Build history of the part. All positions in model axes, mm. A direction names the side the tool comes from. Coordinates: 2 decimals unless noted, no trailing zeros. Order: outer loops, then holes, each group sorted by start corner. A loop starts at its lowest first (then second) coordinate and runs counter-clockwise, first axis right, second up. Notation, with made-up numbers: (-23.5, 58.5) -> (11.5, 58.5) arc R23 cw to (11.5, 76.5) -> close; hole circle Ø6 at (-12.75, 4.25). An arc over 180 degrees is marked (long way). Write each question's results on one line, items separated by ' | '.
from build123d import *

# Parameters (mm, degrees)
SKETCH003_R        = 38.1
PAD003_DEPTH       = 2
SKETCH004_R        = 8
PAD004_DEPTH       = 16
SKETCH005_R        = 38.1
PAD005_DEPTH       = 2
POCKET_DEPTH       = 239.207569
POLARPATTERN_COUNT = 3
SKETCH007_R        = 4
POCKET001_DEPTH    = 20.001


with BuildPart() as part:
    # Sketch003 → Pad003 (new body)
    with BuildSketch(Plane.XY):
        Circle(SKETCH003_R)
    extrude(amount=PAD003_DEPTH)

    # Sketch004 (on Face3 of Pad003) → Pad004 (join)
    with BuildSketch(Plane.XY.offset(2)):
        Circle(SKETCH004_R)
    extrude(amount=PAD004_DEPTH)

    # Sketch005 (on Face5 of Pad004) → Pad005 (join)
    with BuildSketch(Plane.XY.offset(18)):
        Circle(SKETCH005_R)
    extrude(amount=PAD005_DEPTH)

    # Sketch006 (on Face3 of Pad005) → Pocket (cut, through all)
    with BuildSketch(Plane.XY.offset(20)):
        with BuildLine():
            Line((-15, 29.1), (15, 29.1))
            ThreePointArc((15.842922, 27.561965), (15.876937, 28.580606), (15, 29.1))
            Line((15.842922, 27.561965), (6.842922, 13.461965))
            ThreePointArc((6, 13), (6.480606, 13.123063), (6.842922, 13.461965))
            Line((6, 13), (-6, 13))
            ThreePointArc((-6.842922, 13.461965), (-6.480606, 13.123063), (-6, 13))
            Line((-6.842922, 13.461965), (-15.842922, 27.561965))
            ThreePointArc((-15, 29.1), (-15.876937, 28.580606), (-15.842922, 27.561965))
        make_face()
    pocket = extrude(amount=-POCKET_DEPTH, mode=Mode.SUBTRACT)

    # PolarPattern: Pocket ×3 about axis
    polarpattern_axis = Axis((0, 0, 20), (0, 0, 1))
    for i in range(1, POLARPATTERN_COUNT):
        add(pocket.rotate(polarpattern_axis, i * 360 / POLARPATTERN_COUNT), mode=Mode.SUBTRACT)

    # Sketch007 (on Face3 of PolarPattern) → Pocket001 (cut, through all)
    with BuildSketch(Plane.XY.offset(20)):
        Circle(SKETCH007_R)
    extrude(amount=-POCKET001_DEPTH, mode=Mode.SUBTRACT)


with BuildPart() as part_1:
    # Body012 placement: moved
    add(part.part.moved(Location((-81, 129, 44))))


solid = part_1.part
Item 1: Pin check, flat tips, straight feed: pin 1 (10.5 mm diameter, centred on x = -81, y = 129, fed in from -Z); pin 2 (12 mm diameter, centred on y = 99.5, z = 60.5, fed in from -X); pin 3 (6 mm diameter, centred on y = 150, z = 47, fed in from -X); pin 4 (1.6 mm diameter, centred on x = -77.5, z = 63.5, fed in from -Y). Stop position of each tip, or through.
Answer:
pin 1: stops at z = 44 | pin 2: stops at x = -110.84 | pin 3: stops at x = -114.49 | pin 4: stops at y = 91
Item 2: Pull direction X, two halves, no side cores. Call faces 1 (the cylindrical face through (-97.83, 100.96, 45.01)), 2 (the cylindrical face through (-63.42, 95.2, 62.99)), 3 (the flat face through (-82, 121, 44)): released by +X, released by -X, zero draft, split by the parting line, or undercut.
Answer:
face 1: undercut | face 2: split by the parting line | face 3: zero draft
Item 3: Slice it at B-B, the plane y = 161. List the corners of the cut face in (x, z), and give its area (3 significant figures).
Answer:
outline: (-101.68, 44) -> (-60.32, 44) -> (-60.32, 46) -> (-101.68, 46) -> close; (-101.68, 62) -> (-60.32, 62) -> (-60.32, 64) -> (-101.68, 64) -> close | area: 165 mm^2
Item 4: Tool access for faces 4 (the flat face through (-82, 121, 64)), 5 (the cylindrical face through (-82.73, 121.19, 53.89)), 6 (the cylindrical face through (-64.2, 100.96, 63.01)): list every direction of +Z, -Z, +X, -X, +Y, -Y with a clear straight run to the whole face (end or side of a thin tool).
Answer:
face 4: +Z, +X, -X, +Y, -Y | face 5: none | face 6: +Z, -Z
Item 5: Slice it at A-A, the plane x = -81. List the corners of the cut face in (y, z).
Answer:
outline: (90.9, 44) -> (125, 44) -> (125, 64) -> (90.9, 64) -> (90.9, 62) -> (121, 62) -> (121, 46) -> (90.9, 46) -> close; (133, 44) -> (142, 44) -> (142, 46) -> (137, 46) -> (137, 62) -> (142, 62) -> (142, 64) -> (133, 64) -> close; (158.1, 44) -> (167.1, 44) -> (167.1, 46) -> (158.1, 46) -> close; (158.1, 62) -> (167.1, 62) -> (167.1, 64) -> (158.1, 64) -> close
Item 6: Slice it at D-D, the plane y = 147. List the corners of the cut face in (x, z).
Answer:
outline: (-114.58, 44) -> (-90.74, 44) -> (-90.74, 46) -> (-114.58, 46) -> close; (-114.58, 62) -> (-90.74, 62) -> (-90.74, 64) -> (-114.58, 64) -> close; (-71.26, 44) -> (-47.42, 44) -> (-47.42, 46) -> (-71.26, 46) -> close; (-71.26, 62) -> (-47.42, 62) -> (-47.42, 64) -> (-71.26, 64) -> close
Item 7: Slice it at C-C, the plane x = -68. List the corners of the cut face in (y, z).
Answer:
outline: (93.19, 44) -> (107.17, 44) -> (107.17, 46) -> (93.19, 46) -> close; (93.19, 62) -> (107.17, 62) -> (107.17, 64) -> (93.19, 64) -> close; (125.52, 44) -> (152.11, 44) -> (152.11, 46) -> (125.52, 46) -> close; (125.52, 62) -> (152.11, 62) -> (152.11, 64) -> (125.52, 64) -> close; (158.1, 44) -> (164.81, 44) -> (164.81, 46) -> (158.1, 46) -> close; (158.1, 62) -> (164.81, 62) -> (164.81, 64) -> (158.1, 64) -> close
Item 8: Drill centre lines: line 1 (Z direction, x = -115.5, y = 139.5); line 2 (Y direction, x = -81, z = 54.25); line 3 (Y direction, x = -69, z = 63). Where is each one in solid material? Low to high. Write a range as from..to.
Answer:
line 1: z = 44..46, 62..64 | line 2: y = 121..125, 133..137 | line 3: y = 92.84..109.1, 123.78..150.54, 158.1..165.16
